For this review, take the finished solid that the model builds, in its own axes (mm). Coordinates: 2 decimals unless noted, no trailing zeros. Loops run counter-clockwise (first coordinate to the right, second up) from the corner with the lowest first, then second, coordinate; pieces in that order, holes last. Notation, with made-up numbers: M 40,4.5 L 98,4.5 A7 cw 98,16.5 Z; hole C 15,-23 d7. An arc over 180 degrees is marked long. Answer as a JSON object with one key per item and string values. Group by question number.
Item 1: Add section B-B (y = 30). State the section outline as (x, z) points, then the cut area to 3 significant figures.
Item 2: Add section D-D (z = 1). Count the separate pieces of the cut face and the enclosed holes in it, then the cut area to 3 significant figures.
Item 3: Add section C-C (x = -35). State the section outline as (y, z) points, then the cut area to 3 significant figures.
Item 4: Wall thickness on L1, parallel to Y at x = -33.5, z = 4.75; L2, parallel to Y at x = 5, z = 5.1; L3, parallel to X at y = 37, z = 2.85: over which ranges is each line inside the solid? List them lowest first. Write a range as from..to.
Item 5: Add section A-A (y = 92). State the section outline as (x, z) points.
Item 6: Insertion check: pin 1 (6 mm diameter, centred on x = -24.75, y = 75.25, fed in from +Z); pin 2 (3 mm diameter, centred on y = 24, z = 3.5, fed in from -X); pin 3 (1.8 mm diameter, centred on x = -15, z = 4, fed in from -Y). Each pin has a flat end and moves straight along its axis. Give the tip position at first contact, or say it passes through.
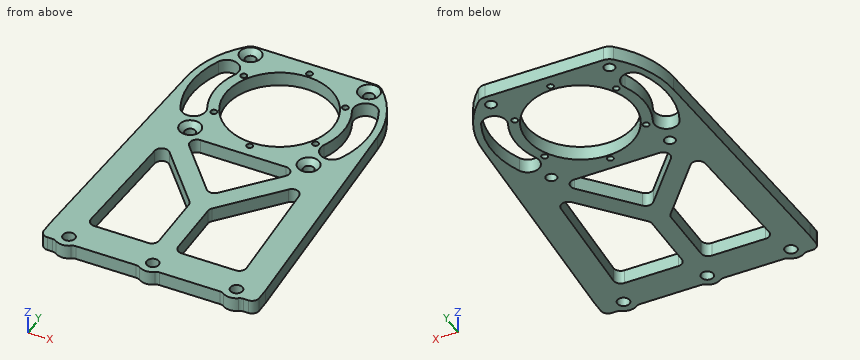
from build123d import *

# Parameters (mm, degrees)
SKETCH_1_W                   = 90
SKETCH_1_H                   = 8
SKETCH_1_R                   = 2.1
SKETCH_1_R_2                 = 1.3
SKETCH_1_R_3                 = 22.5
EXTRUDE_1_DEPTH              = 6
HOLE_WIZARD_M4_1_D           = 4.5
HOLE_WIZARD_M4_1_DEPTH       = 11.4
HOLE_WIZARD_M4_1_CSINK_D     = 8.96
HOLE_WIZARD_M4_1_CSINK_ANGLE = 90
HOLE_WIZARD_M4_1_TIP         = 1.351936393
SKETCH_4_R                   = 2.55
CUT_EXTRUDE_1_DEPTH          = 148.17676447
EXTRUDE_2_DEPTH              = 6
CUT_EXTRUDE_3_DEPTH          = 148.17676447
FILLET_1_R                   = 5
FILLET_2_R                   = 3
FILLET_4_R                   = 3
CUT_EXTRUDE_4_DEPTH          = 138.461757743


with BuildPart() as part:
    # 草图1 → 凸台-拉伸1 (new body)
    # profile 1 of 3: a face of its own
    with BuildSketch(Plane.XY):
        with BuildLine():
            Line((-39.951065042, 101.977979269), (-45, 0))
            Line((-45, 0), (45, 0))
            Line((45, 0), (39.951065042, 101.977979269))
            ThreePointArc((39.951065042, 101.977979269), (39.987764389, 100.989292249), (40, 100))
            ThreePointArc((40, 100), (-0.989292249, 60.012235611), (-39.951065042, 101.977979269))
        make_face()
    # profile 2 of 3: a face of its own
    with BuildSketch(Plane.XY):
        with Locations((0, -4)):
            Rectangle(SKETCH_1_W, SKETCH_1_H)
    # profile 3 of 3: a face of its own
    with BuildSketch(Plane.XY):
        with BuildLine():
            ThreePointArc((39.951065042, 101.977979269), (0, 140), (-39.951065042, 101.977979269))
            ThreePointArc((-39.951065042, 101.977979269), (-0.989292249, 60.012235611), (40, 100))
            ThreePointArc((40, 100), (39.987764389, 100.989292249), (39.951065042, 101.977979269))
        make_face()
        with Locations((-24.748737342, 75.251262658)):
            Circle(SKETCH_1_R, mode=Mode.SUBTRACT)
        with Locations((-21.217622393, 87.75)):
            Circle(SKETCH_1_R_2, mode=Mode.SUBTRACT)
        with Locations((-24.748737342, 124.748737342)):
            Circle(SKETCH_1_R, mode=Mode.SUBTRACT)
        with Locations((-21.217622393, 112.25)):
            Circle(SKETCH_1_R_2, mode=Mode.SUBTRACT)
        with Locations((0, 75.5)):
            Circle(SKETCH_1_R_2, mode=Mode.SUBTRACT)
        with Locations((0, 100)):
            Circle(SKETCH_1_R_3, mode=Mode.SUBTRACT)
        with Locations((21.217622393, 87.75)):
            Circle(SKETCH_1_R_2, mode=Mode.SUBTRACT)
        with Locations((24.748737342, 75.251262658)):
            Circle(SKETCH_1_R, mode=Mode.SUBTRACT)
        with Locations((21.217622393, 112.25)):
            Circle(SKETCH_1_R_2, mode=Mode.SUBTRACT)
        with Locations((0, 124.5)):
            Circle(SKETCH_1_R_2, mode=Mode.SUBTRACT)
        with Locations((24.748737342, 124.748737342)):
            Circle(SKETCH_1_R, mode=Mode.SUBTRACT)
    extrude(amount=EXTRUDE_1_DEPTH)

    # M4 六角凹锥坑螺钉的锥形沉头孔1
    with Locations(Plane.XY.offset(6)):
        with Locations((-24.748737342, 124.748737342), (24.748737342, 124.748737342), (24.748737342, 75.251262658), (-24.748737342, 75.251262658)):
            CounterSinkHole(HOLE_WIZARD_M4_1_D / 2, HOLE_WIZARD_M4_1_CSINK_D / 2, depth=HOLE_WIZARD_M4_1_DEPTH, counter_sink_angle=HOLE_WIZARD_M4_1_CSINK_ANGLE)
            with Locations((0, 0, -(HOLE_WIZARD_M4_1_DEPTH + HOLE_WIZARD_M4_1_TIP / 2))):  # 118° drill point
                Cone(0, HOLE_WIZARD_M4_1_D / 2, HOLE_WIZARD_M4_1_TIP, mode=Mode.SUBTRACT)

    # 草图4 → 切除-拉伸1 (cut, through all)
    with BuildSketch(Plane.XY.offset(6)):
        with Locations((-35, -4)):
            Circle(SKETCH_4_R)
        with Locations((0, -4)):
            Circle(SKETCH_4_R)
        with Locations((35, -4)):
            Circle(SKETCH_4_R)
    extrude(amount=-CUT_EXTRUDE_1_DEPTH, mode=Mode.SUBTRACT)

    # 草图5 → 凸台-拉伸2 (add)
    with BuildSketch(Plane.XY.offset(6)):
        with BuildLine():
            ThreePointArc((-38.847401721, -8), (-35, -9.55), (-31.152598279, -8))
            Line((-31.152598279, -8), (-38.847401721, -8))
        make_face()
        with BuildLine():
            ThreePointArc((-3.847401721, -8), (0, -9.55), (3.847401721, -8))
            Line((3.847401721, -8), (-3.847401721, -8))
        make_face()
        with BuildLine():
            ThreePointArc((31.152598279, -8), (35, -9.55), (38.847401721, -8))
            Line((38.847401721, -8), (31.152598279, -8))
        make_face()
    extrude(amount=-EXTRUDE_2_DEPTH)

    # 草图6 → 切除-拉伸3 (cut, through all)
    with BuildSketch(Plane.XY.offset(6)):
        with BuildLine():
            ThreePointArc((26.739720017, 129.748737342), (0, 140), (-26.739720017, 129.748737342))
            Line((-26.739720017, 129.748737342), (26.739720017, 129.748737342))
        make_face()
        Polygon((32.688241225, 6), (29.805909331, 64.217106098), (4, 34.505425616), (4, 6), align=None)
        Polygon((-4, 34.505425616), (-29.805909331, 64.217106098), (-32.688241225, 6), (-4, 6), align=None)
        Polygon((24.450633349, 70.251262658), (-24.450633349, 70.251262658), (0, 42.099981634), align=None)
    extrude(amount=-CUT_EXTRUDE_3_DEPTH, mode=Mode.SUBTRACT)

    # 圆角1
    fillet_1_edges = [part.edges().sort_by_distance(p)[0] for p in [
        (-26.739720017, 129.748737342, 3),
        (26.739720017, 129.748737342, 3),
    ]]
    fillet(fillet_1_edges, radius=FILLET_1_R)

    # 圆角2
    fillet_2_edges = [part.edges().sort_by_distance(p)[0] for p in [
        (24.450633349, 70.251262658, 3),
        (0, 42.099981634, 3),
        (-24.450633349, 70.251262658, 3),
        (-4, 34.505425616, 3),
        (-4, 6, 3),
        (-32.688241225, 6, 3),
        (-29.805909331, 64.217106098, 3),
        (4, 34.505425616, 3),
        (29.805909331, 64.217106098, 3),
        (32.688241225, 6, 3),
        (4, 6, 3),
    ]]
    fillet(fillet_2_edges, radius=FILLET_2_R)

    # 圆角4
    fillet_4_edges = [part.edges().sort_by_distance(p)[0] for p in [
        (-38.847401721, -8, 3),
        (-31.152598279, -8, 3),
        (-3.847401721, -8, 3),
        (3.847401721, -8, 3),
        (31.152598279, -8, 3),
        (38.847401721, -8, 3),
        (45, 0, 3),
        (45, -8, 3),
        (-45, -8, 3),
        (-45, 0, 3),
    ]]
    fillet(fillet_4_edges, radius=FILLET_4_R)

    # 草图7 → 切除-拉伸4 (cut, through all)
    with BuildSketch(Plane.XY.offset(6)):
        with BuildLine():
            ThreePointArc((33.53338812, 84.363124316), (37, 100), (33.53338812, 115.636875684))
            ThreePointArc((33.53338812, 115.636875684), (26.888757876, 118.055323311), (24.47031025, 111.410693067))
            ThreePointArc((24.47031025, 111.410693067), (27, 100), (24.47031025, 88.589306933))
            ThreePointArc((24.47031025, 88.589306933), (26.888757876, 81.944676689), (33.53338812, 84.363124316))
        make_face()
        with BuildLine():
            ThreePointArc((-33.53338812, 84.363124316), (-37, 100), (-33.53338812, 115.636875684))
            ThreePointArc((-33.53338812, 115.636875684), (-26.888757876, 118.055323311), (-24.47031025, 111.410693067))
            ThreePointArc((-24.47031025, 111.410693067), (-27, 100), (-24.47031025, 88.589306933))
            ThreePointArc((-24.47031025, 88.589306933), (-26.888757876, 81.944676689), (-33.53338812, 84.363124316))
        make_face()
    extrude(amount=-CUT_EXTRUDE_4_DEPTH, mode=Mode.SUBTRACT)


solid = part.part
From the geometry:
{
 "1": {"outline": "M -43.51,0 L -31.5,0 L -31.5,6 L -43.51,6 Z; M -4,0 L 4,0 L 4,6 L -4,6 Z; M 31.5,0 L 43.51,0 L 43.51,6 L 31.5,6 Z", "area": "192 mm²"},
 "2": {"separate pieces": "1", "enclosed holes": "19", "area": "5,880 mm²"},
 "3": {"outline": "M -9.55,0 L -6.55,0 L -6.55,6 L -9.55,6 Z; M -1.45,0 L 88,0 L 88,6 L -1.45,6 Z; M 112,0 L 119.36,0 L 119.36,6 L 112,6 Z", "area": "599 mm²"},
 "4": {"L1": "y = -9.34..-6.06, -1.94..84.29, 115.71..121.86", "L2": "y = -8..6.76, 35.66..47.86, 70.25..78.06, 121.94..129.75", "L3": "x = -43.17..-31.15, -6.17..6.17, 31.15..43.17"},
 "5": {"outline": "M -40.45,0 L -36.12,0 L -36.12,6 L -40.45,6 Z; M -25.79,0 L -21.03,0 L -21.03,6 L -25.79,6 Z; M 21.03,0 L 25.79,0 L 25.79,6 L 21.03,6 Z; M 36.12,0 L 40.45,0 L 40.45,6 L 36.12,6 Z"},
 "6": {"pin 1": "stops at z = 4.52", "pin 2": "stops at x = -43.89", "pin 3": "stops at y = -8"}
}
